Build history of the part. All positions in model axes, mm. Face numbers are marked on the shaded views. A direction names the side the tool comes from. Round coordinates to 2 decimals unless told otherwise and drop trailing zeros. Write each loop counter-clockwise with the first axis right and the second up, starting at its lowest first coordinate (ties: lowest second). Pieces come first, ordered by that corner, then holes.
Item 1: Drop flat-ended pins along their axis: pin 1 Ø9 at (y, z) = (21.5, 7.5) entering from -X; pin 2 Ø3 at (y, z) = (4, 14) entering from -X; pin 3 Ø9 at (x, z) = (19.5, 10) entering from +Y; pin 4 Ø9 at (x, z) = (34, 7.5) entering from -Y. Give the stop position or say it passes through.
Item 2: 3-axis set-ups, long thin cutter, end or side, ignore diameter. For the marked faces 1, 2 and 3: which of +Z, -Z, +X, -X, +Y, -Y reach the whole face in a straight line?
Item 3: Band-saw the part on D-D, the plane z = 14. Write the cut outline in (x, y).
Item 4: Band-saw the part on A-A, the plane y = 26. Write the cut outline in (x, z), then the cut area to 3 significant figures.
Item 5: Wall check: probe 1 along Y at (x, z) = (17, 16.5); probe 2 along X at (y, z) = (31.5, 16); probe 3 along Y at (x, z) = (1.35, 14). Give the ranges that are in metal, low to high.
Item 6: Band-saw the part on B-B, the plane y = 4. Write the cut outline in (x, z).
Item 7: Band-saw the part on C-C, the plane z = 9. Write the cut outline in (x, y).
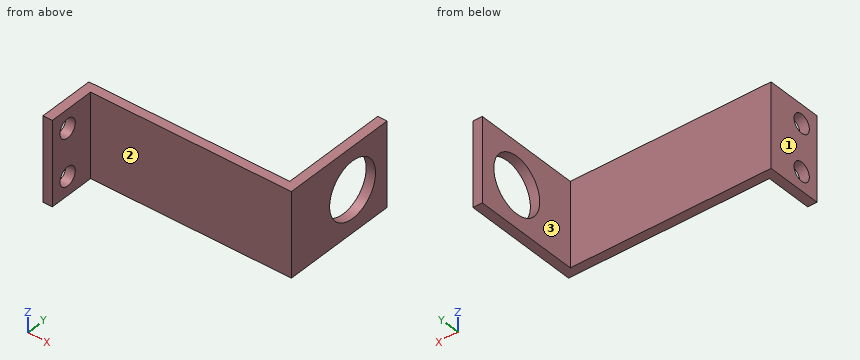
```python
from build123d import *

# Parameters (mm, degrees)
BOSS_EXTRUDE1_DEPTH = 18
CUT_EXTRUDE1_REACH  = 47
SKETCH2_R           = 2
CUT_EXTRUDE2_REACH  = 4
SKETCH3_R           = 6


with BuildPart() as part:
    # Sketch1 → Boss-Extrude1 (new body)
    with BuildSketch(Plane.XY):
        Polygon((0, 0), (0, 12), (43, 12), (43, 35), (45, 35), (45, 10), (2, 10), (2, 0), align=None)
    extrude(amount=BOSS_EXTRUDE1_DEPTH)

    # Sketch2 → Cut-Extrude1 (cut, up to next)
    with BuildSketch(Plane.ZY, mode=Mode.PRIVATE) as cut_extrude1_sk1:
        with Locations((4, 4)):
            Circle(SKETCH2_R)
    cut_extrude1_tool1 = extrude(cut_extrude1_sk1.sketch, amount=-CUT_EXTRUDE1_REACH, mode=Mode.PRIVATE) & part.part
    add(cut_extrude1_tool1.solids().sort_by_distance((0, 4, 4))[0], mode=Mode.SUBTRACT)
    # Sketch2 → Cut-Extrude1 (cut, up to next)
    with BuildSketch(Plane.ZY, mode=Mode.PRIVATE) as cut_extrude1_sk2:
        with Locations((14, 4)):
            Circle(SKETCH2_R)
    cut_extrude1_tool2 = extrude(cut_extrude1_sk2.sketch, amount=-CUT_EXTRUDE1_REACH, mode=Mode.PRIVATE) & part.part
    add(cut_extrude1_tool2.solids().sort_by_distance((0, 4, 14))[0], mode=Mode.SUBTRACT)

    # Sketch3 → Cut-Extrude2 (cut, up to next)
    with BuildSketch(Plane.ZY.offset(-43), mode=Mode.PRIVATE) as cut_extrude2_sk1:
        with Locations((9, 26)):
            Circle(SKETCH3_R)
    cut_extrude2_tool1 = extrude(cut_extrude2_sk1.sketch, amount=-CUT_EXTRUDE2_REACH, mode=Mode.PRIVATE) & part.part
    add(cut_extrude2_tool1.solids().sort_by_distance((43, 26, 9))[0], mode=Mode.SUBTRACT)


solid = part.part
```
Results:
1. pin 1: stops at x = 43
1. pin 2: passes through
1. pin 3: stops at y = 12
1. pin 4: stops at y = 10
2. face 1: +Z, -Z, -X, +Y, -Y
2. face 2: +Z, -Z, +X, -Y
2. face 3: +Z, -Z, -X, +Y
3. outline: (0, 0) - (2, 0) - (2, 2) - (0, 2) - close; (0, 6) - (2, 6) - (2, 10) - (45, 10) - (45, 22.68) - (43, 22.68) - (43, 12) - (0, 12) - close; (43, 29.32) - (45, 29.32) - (45, 35) - (43, 35) - close
4. outline: (43, 0) - (45, 0) - (45, 3) - (43, 3) - close; (43, 15) - (45, 15) - (45, 18) - (43, 18) - close
4. area: 12.0 mm2
5. probe 1: y = 10 to 12
5. probe 2: x = 43 to 45
5. probe 3: y = 0 to 2, 6 to 12
6. outline: (0, 0) - (2, 0) - (2, 2) - (0, 2) - close; (0, 6) - (2, 6) - (2, 12) - (0, 12) - close; (0, 16) - (2, 16) - (2, 18) - (0, 18) - close
7. outline: (0, 0) - (2, 0) - (2, 10) - (45, 10) - (45, 20) - (43, 20) - (43, 12) - (0, 12) - close; (43, 32) - (45, 32) - (45, 35) - (43, 35) - close
